For this review, use the dimensioned drawing (mm, ordinates from the lowest corner) and the shaded views. Coordinates: 2 decimals unless noted, no trailing zeros. Loops run counter-clockwise (first coordinate to the right, second up) from the corner with the lowest first, then second, coordinate; pieces in that order, holes last.
1. Take a section at B-B, the plane y = 8.75. State the section outline as (x, z) points (3 decimals).
2. Take a section at A-A, the plane x = 10.16. State the section outline as (y, z) points (3 decimals).
3. To check wall thickness, follow probe 1 along Z at (x, y) = (40, 1.75); probe 2 along X at (y, z) = (11.75, 41.5); probe 3 along X at (y, z) = (2, 9.5). State the ranges of each line that lie inside material, in increasing order.
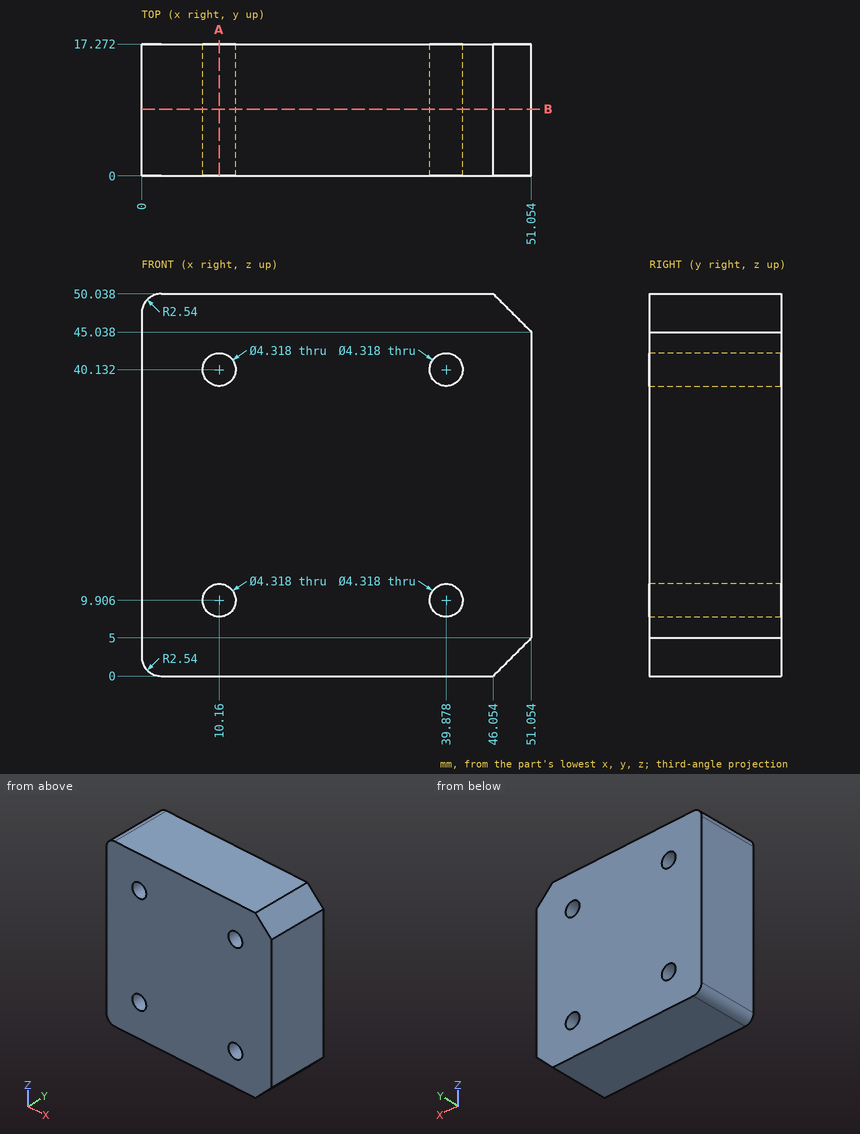
Results list:
1. outline: (0, 2.54) arc R2.54 ccw to (2.54, 0) - (46.054, 0) - (51.054, 5) - (51.054, 45.038) - (46.054, 50.038) - (2.54, 50.038) arc R2.54 ccw to (0, 47.498) - close; hole circle Ø4.318 at (10.16, 9.906); hole circle Ø4.318 at (10.16, 40.132); hole circle Ø4.318 at (39.878, 9.906); hole circle Ø4.318 at (39.878, 40.132)
2. outline: (0, 0) - (17.272, 0) - (17.272, 7.747) - (0, 7.747) - close; (0, 12.065) - (17.272, 12.065) - (17.272, 37.973) - (0, 37.973) - close; (0, 42.291) - (17.272, 42.291) - (17.272, 50.038) - (0, 50.038) - close
3. probe 1: z = 0 to 7.75, 12.06 to 37.98, 42.29 to 50.04
3. probe 2: x = 0 to 8.49, 11.83 to 38.21, 41.55 to 51.05
3. probe 3: x = 0 to 8.04, 12.28 to 37.76, 42 to 51.05
